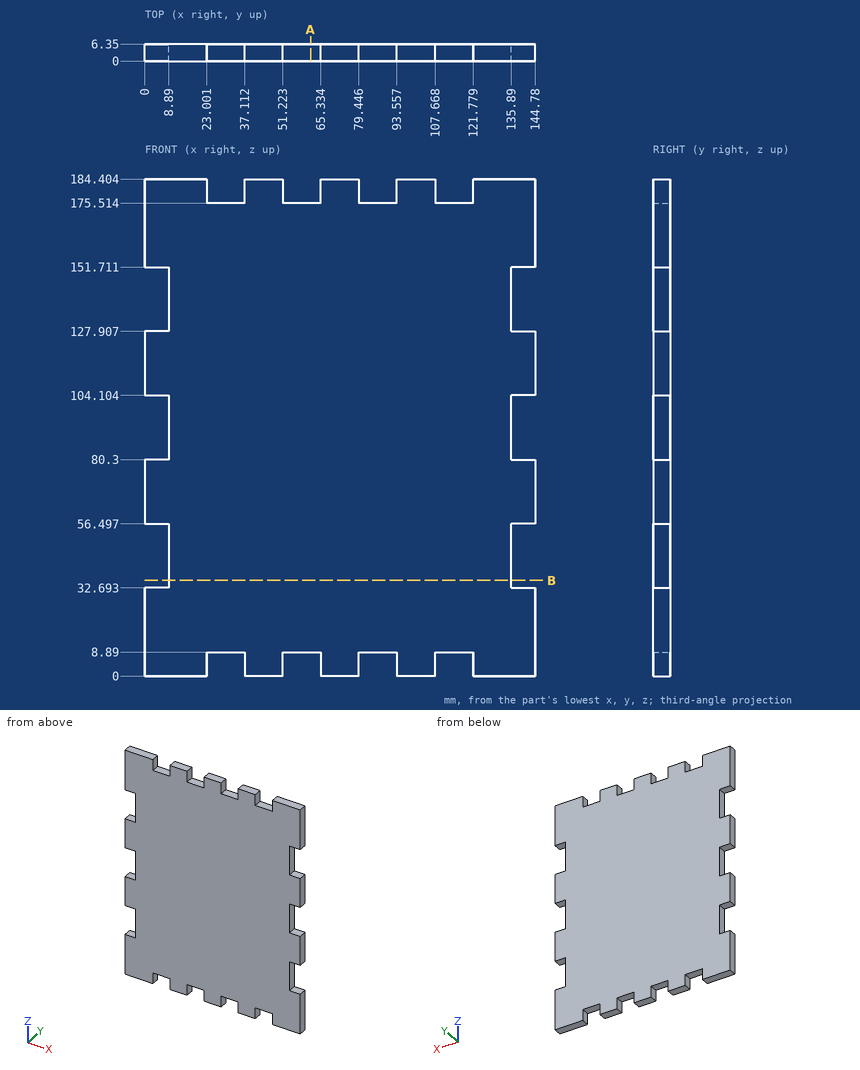
The drawing under review shows one solid part. Ordinate dimensions are in mm from its lowest x, y, z. Coordinates: 2 decimals unless noted, no trailing zeros. Order: outer loops, then holes, each group sorted by start corner. A loop starts at its lowest first (then second) coordinate and runs counter-clockwise, first axis right, second up. Notation, with made-up numbers: (70, 41.5) -> (117, 41.5) arc R16 cw to (117, 50.5) -> close; hole circle Ø5 at (80, 35.5). An arc over 180 degrees is marked (long way). Answer as CSV lines item,"result".
Q1. We need section B-B (z = 35.5). State the section outline as (x, y) points.
Model answer:
outline,"(8.89, 0) -> (135.89, 0) -> (135.89, 6.35) -> (8.89, 6.35) -> close"
Q2. Wall thickness on line 1 along Z through (x, y) = (24, 3.75); line 2 along X through (y, z) = (5.5, 142): over which ranges is each line inside the solid? List them lowest first. Write a range as [from, to].
Model answer:
line 1,"z = [8.89, 175.51]"
line 2,"x = [8.89, 135.89]"
Q3. Clearance check with flat-ended pins moving along their axes: pin 1 Ø3 at (x, y) = (113.5, 4) entering from +Z; pin 2 Ø1.9 at (x, y) = (32, 2.5) entering from -Z; pin 3 Ø1 at (y, z) = (1, 136.5) entering from -X. State where each tip first meets the part, or that it passes through.
Model answer:
pin 1,"stops at z = 175.51"
pin 2,"stops at z = 8.89"
pin 3,"stops at x = 8.89"
Q4. We need section A-A (x = 61.5). State the section outline as (y, z) points.
Model answer:
outline,"(0, 8.89) -> (6.35, 8.89) -> (6.35, 175.51) -> (0, 175.51) -> close"
